Source: three-view drawing plus pictorial views. Frame: mm from the lowest corner of the part. Give positions to 0.01 mm unless a question says otherwise; leave off trailing zeros. Loops run counter-clockwise (first coordinate to the right, second up) from the corner with the lowest first, then second, coordinate; pieces in that order, holes last. Notation, with made-up numbers: M 89.5,40 L 105.5,40 A16 cw 105.5,45 Z; hole C 45.5,45 d5. An arc over 180 degrees is marked long. Answer as a JSON object with one key per item and string values. Group by question number.
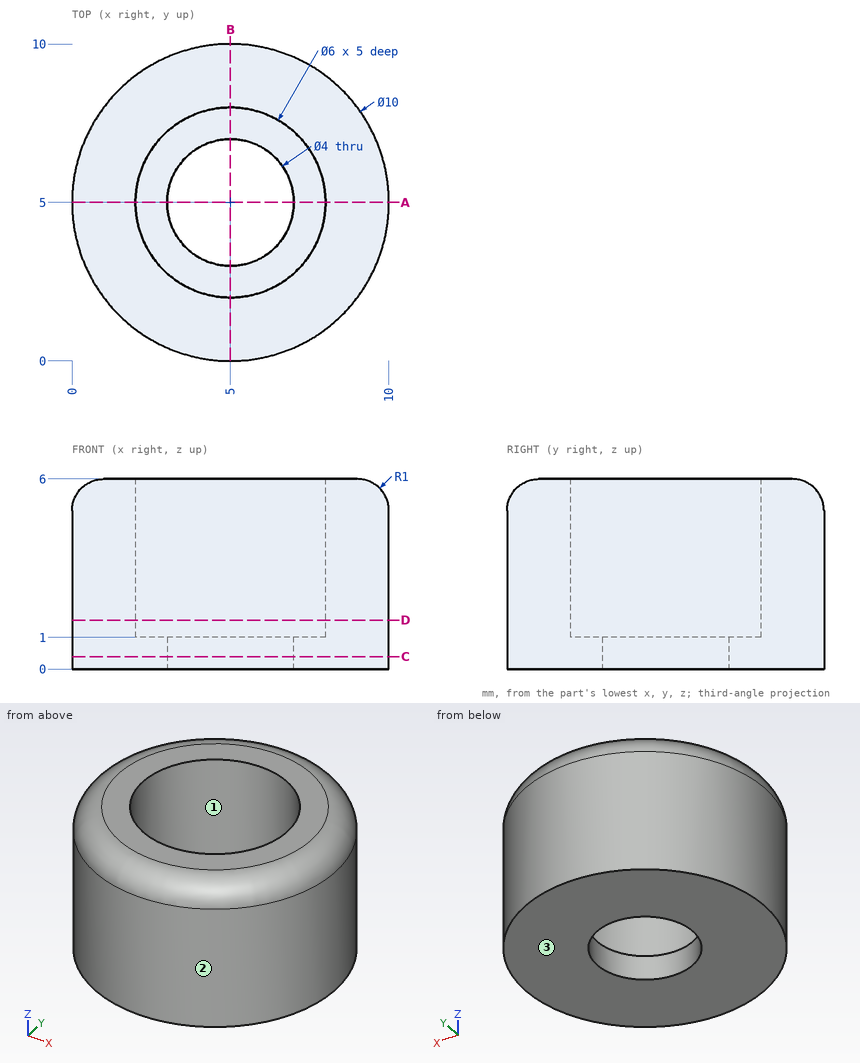
1. Section D-D (z = 1.55). Output: boundary loops of the cut face in (x, y).
2. Mould query, pull axis Y, two halves, no side actions, for the marked faces 1, 2 and 3. Classes: pulls with the +Y half, pulls with the -Y half, needs draft (parallel to the pull), parting line crosses it, or undercut.
3. Section C-C (z = 0.4). Output: boundary loops of the cut face in (x, y).
4. Section A-A (y = 5). Output: boundary loops of the cut face in (x, z).
5. First-contact query: P1, Ø1, axis at x = 7, z = 3.5, coming from the -Y side; P2, Ø1.5, axis at y = 8, z = 5.5, coming from the -X side; P3, Ø1, axis at x = 1.5, z = 4, coming from the -Y side. Flat tips, straight axial feed; report the tip coordinate or a pass-through.
6. Material intervals for L1, parallel to Y at x = 5, z = 2.65; L2, parallel to Z at x = 2.75, y = 6; L3, parallel to Y at x = 7, z = 4.55, sorted ascending.
Geometry results:
{
 "1": {"outline": "C 5,5 d10; hole C 5,5 d6"},
 "2": {"face 1": "undercut", "face 2": "parting line crosses it", "face 3": "needs draft"},
 "3": {"outline": "C 5,5 d10; hole C 5,5 d4"},
 "4": {"outline": "M 0,0 L 3,0 L 3,1 L 2,1 L 2,6 L 1,6 A1 ccw 0,5 Z; M 7,0 L 10,0 L 10,5 A1 ccw 9,6 L 8,6 L 8,1 L 7,1 Z"},
 "5": {"P1": "y = 0.23", "P2": "x = 0.59", "P3": "y = 1"},
 "6": {"L1": "0 to 2, 8 to 10", "L2": "0 to 1", "L3": "0.42 to 2.76, 7.24 to 9.58"}
}
